from build123d import *

# Parameters (mm, degrees)
EXTRUDE_1_DEPTH     = 3
SKETCH_2_R          = 1.575
CUT_EXTRUDE_1_DEPTH = 69.883960397
FILLET_1_R          = 5


with BuildPart() as part:
    # 草图1 → 凸台-拉伸1 (new body)
    with BuildSketch(Plane.XY):
        Polygon((0, 0), (20, 0), (40, -36), (40, -56), (-20, -56), (-20, -36), align=None)
    extrude(amount=EXTRUDE_1_DEPTH)

    # 草图2 → 切除-拉伸1 (cut, through all)
    with BuildSketch(Plane.XY.offset(3)):
        with Locations((-15, -41)):
            Circle(SKETCH_2_R)
        with Locations(Location((-5, -41, 0), (0, 0, 180))):
            Circle(SKETCH_2_R)
        with Locations((-5, -51)):
            Circle(SKETCH_2_R)
        with Locations(Location((-15, -51, 0), (0, 0, 180))):
            Circle(SKETCH_2_R)
        with Locations((35, -51)):
            Circle(SKETCH_2_R)
        with Locations(Location((25, -51, 0), (0, 0, 180))):
            Circle(SKETCH_2_R)
        with Locations((25, -41)):
            Circle(SKETCH_2_R)
        with Locations(Location((35, -41, 0), (0, 0, 180))):
            Circle(SKETCH_2_R)
        with Locations((10, -25)):
            Circle(SKETCH_2_R)
        with Locations((10, -5)):
            Circle(SKETCH_2_R)
        with Locations((10, -45)):
            Circle(SKETCH_2_R)
        Polygon((0, -12.354756169), (-9.802913239, -30), (0, -30), align=None)
        Polygon((29.802913239, -30), (20, -30), (20, -12.354756169), align=None)
    extrude(amount=-CUT_EXTRUDE_1_DEPTH, mode=Mode.SUBTRACT)

    # 圆角1
    fillet_1_edges = [part.edges().sort_by_distance(p)[0] for p in [
        (0, 0, 1.5),
        (20, 0, 1.5),
        (40, -36, 1.5),
        (40, -56, 1.5),
        (-20, -56, 1.5),
        (-20, -36, 1.5),
    ]]
    fillet(fillet_1_edges, radius=FILLET_1_R)


solid = part.part
Input: part model. Units: mm. Frame: model coordinates. A direction names the side the tool comes from. Give positions to 0.01 mm unless a question says otherwise; leave off trailing zeros. Loops run counter-clockwise (first coordinate to the right, second up) from the corner with the lowest first, then second, coordinate; pieces in that order, holes last. Notation, with made-up numbers: (41.25, 62) - (93.25, 62) arc R13 ccw to (93.25, 75) - close; hole circle Ø4 at (60, 86.5). An arc over 180 degrees is marked (long way). Use CSV: the item, a comma, the result in double quotes. Start each with the question number.
Item 1: Line query: line 1 (Y direction, x = -5, z = 1.35) (3 decimals); line 2 (X direction, y = -40, z = 1.95); line 3 (X direction, y = -23, z = 2.45). Output: solid intervals per line, ascending.
Item 2: Section A-A on x = 10. Return loops of the section in (y, z) (3 decimals), then the cut area to 3 significant figures.
Item 3: Reachability of faces 1 (the flat face through (-5, -30, 2)), 2 (the flat face through (-20, -44, 1)) from +Z, -Z, +X, -X, +Y, -Y: full face, straight path, thin tool, end or side. Return the list, or none.
Item 4: Section B-B on z = 1.85. State how many separate pieces and enclosed holes the cut face has, then the cut area to 3 significant figures.
Item 5: Section D-D on y = -25. Return loops of the section in (x, z) (3 decimals), then the cut area to 3 significant figures.
Item 6: Mould query, pull axis Y, two halves, no side actions, for faces 3 (the flat face through (40, -44, 1)), 4 (the cylindrical face through (23.839, -39.936, 1.521)), 5 (the cylindrical face through (26.161, -52.064, 1.521)), 6 (the cylindrical face through (39.836, -36.024, 1.521)). Classes: pulls with the +Y half, pulls with the -Y half, needs draft (parallel to the pull), parting line crosses it, or undercut.
Item 7: Contact query for flat-ended pins moving along their axis: P1, Ø3, axis at x = 10, y = -45, coming from the +Z side; P2, Ø1.5, axis at y = -12, z = 0.5, coming from the -X side. Output: stop coordinate, or through.
Item 8: Section C-C on y = -5. Return loops of the section in (x, z) (3 decimals), then the cut area to 3 significant figures.
Ans:
1,line 1,"y = -56 to -52.575, -49.425 to -42.575, -39.425 to -30, -21.355 to -9"
1,line 2,"x = -20 to -16.22, -13.78 to -6.22, -3.78 to 23.78, 26.22 to 33.78, 36.22 to 40"
1,line 3,"x = -12.78 to -5.91, 0 to 20, 25.91 to 32.78"
2,outline,"(-56, 0) - (-46.575, 0) - (-46.575, 3) - (-56, 3) - close; (-43.425, 0) - (-26.575, 0) - (-26.575, 3) - (-43.425, 3) - close; (-23.425, 0) - (-6.575, 0) - (-6.575, 3) - (-23.425, 3) - close; (-3.425, 0) - (0, 0) - (0, 3) - (-3.425, 3) - close"
2,area,"140 mm2"
3,face 1,"+Z, -Z"
3,face 2,"+Z, -Z, -X, +Y, -Y"
4,separate pieces,"1"
4,enclosed holes,"13"
4,area,"2,370 mm2"
5,outline,"(-13.889, 0) - (-7.025, 0) - (-7.025, 3) - (-13.889, 3) - close; (0, 0) - (8.425, 0) - (8.425, 3) - (0, 3) - close; (11.575, 0) - (20, 0) - (20, 3) - (11.575, 3) - close; (27.025, 0) - (33.889, 0) - (33.889, 3) - (27.025, 3) - close"
5,area,"91.7 mm2"
6,face 3,"needs draft"
6,face 4,"undercut"
6,face 5,"undercut"
6,face 6,"pulls with the +Y half"
7,P1,"passes through"
7,P2,"stops at x = -7.08"
8,outline,"(-2.778, 0) - (8.425, 0) - (8.425, 3) - (-2.778, 3) - close; (11.575, 0) - (22.778, 0) - (22.778, 3) - (11.575, 3) - close"
8,area,"67.2 mm2"
